from build123d import *

# Parameters (mm, degrees)
F0_R     = 11.3
F1_DEPTH = 35
F2_SIZE  = 1
F3_R     = 7.3
F4_DEPTH = 76.5
F5_SIZE2 = 20
F5_SIZE  = 2
F6_R     = 3.75
F7_DEPTH = 111.501
F8_SIZE  = 1


with BuildPart() as f1:
    # F0 (on Front) → F1 (new body)
    with BuildSketch(Plane.XZ):
        Circle(F0_R)
    extrude(amount=-F1_DEPTH)

    # F2
    f2_edges = [f1.edges().sort_by_distance(p)[0] for p in [
        (-11.3, 0, 0),
    ]]
    chamfer(f2_edges, length=F2_SIZE)

    # F3 (on face) → F4 (join)
    with BuildSketch(Plane(origin=(0, 35, 0), x_dir=(-1, 0, 0), z_dir=(0, 1, 0))):
        Circle(F3_R)
    extrude(amount=F4_DEPTH)

    # F5
    f5_edges = [f1.edges().sort_by_distance(p)[0] for p in [
        (7.3, 111.5, 0),
    ]]
    f5_side = f1.faces().sort_by_distance((0, 111.5, 0))[0]
    chamfer(f5_edges, length=F5_SIZE, length2=F5_SIZE2, reference=f5_side)

    # F6 (on face) → F7 (cut, through all)
    with BuildSketch(Plane.XZ):
        Circle(F6_R)
    extrude(amount=-F7_DEPTH, mode=Mode.SUBTRACT)

    # F8
    f8_edges = [f1.edges().sort_by_distance(p)[0] for p in [
        (-11.3, 35, 0),
    ]]
    chamfer(f8_edges, length=F8_SIZE)


solid = f1.part
Input: part model. Units: mm. Frame: model coordinates. A direction names the side the tool comes from. Coordinates: 2 decimals unless noted, no trailing zeros. Loops run counter-clockwise (first coordinate to the right, second up) from the corner with the lowest first, then second, coordinate; pieces in that order, holes last. Notation, with made-up numbers: (38, -11) -> (68, -11) arc R29 ccw to (68, 27) -> close; hole circle Ø8 at (37, 63.25). An arc over 180 degrees is marked (long way). One line per item, written item: value.
(1) Cut plane A-A (z = 0). Output: boundary loops of the cut face in (x, y).
Answer below:
outline: (-11.3, 1) -> (-10.3, 0) -> (-3.75, 0) -> (-3.75, 111.5) -> (-5.3, 111.5) -> (-7.3, 91.5) -> (-7.3, 35) -> (-10.3, 35) -> (-11.3, 34) -> close; (3.75, 0) -> (10.3, 0) -> (11.3, 1) -> (11.3, 34) -> (10.3, 35) -> (7.3, 35) -> (7.3, 91.5) -> (5.3, 111.5) -> (3.75, 111.5) -> close
(2) Pin query (flat end, axial travel): pin 1 Ø6 at (x, y) = (-8.5, 74) entering from -Z; pin 2 Ø1 at (y, z) = (85, -6) entering from -X; pin 3 Ø3 at (y, z) = (29.5, 4) entering from -X; pin 4 Ø12 at (x, z) = (0, 0) entering from +Y. Return the tip coordinate at first contact, or that it passes through.
Answer below:
pin 1: stops at z = -4.8
pin 2: stops at x = -4.8
pin 3: stops at x = -11.02
pin 4: stops at y = 111.5
(3) Draft query along X for faces 1 (the face through (-1, 111.5, 4)), 2 (the face through (-6.963, 62.854, 2.193)), 3 (the face through (-3.746, 54.97, 0.165)). Return one class per face: pulls with the +X half, pulls with the -X half, needs draft (parallel to the pull), parting line crosses it, or undercut.
Answer below:
face 1: needs draft
face 2: parting line crosses it
face 3: undercut
(4) Set-up query: faces 4 (the face through (0, 0, -4)), 5 (the face through (4, 35, -7)). Return all of +Z, -Z, +X, -X, +Y, -Y with unobstructed straight access to the full face (end or side cutting, diameter ignored); none if empty.
Answer below:
face 4: +Z, -Z, +X, -X, -Y
face 5: +Y
(5) Cut plane D-D (y = 43). Output: boundary loops of the cut face in (x, z), then the cut area to 3 significant figures.
Answer below:
outline: circle Ø14.6 at (0, 0); hole circle Ø7.5 at (0, 0)
area: 123 mm2
(6) Cut plane B-B (x = 0). Output: boundary loops of the cut face in (y, z).
Answer below:
outline: (0, -10.3) -> (1, -11.3) -> (34, -11.3) -> (35, -10.3) -> (35, -7.3) -> (91.5, -7.3) -> (111.5, -5.3) -> (111.5, -3.75) -> (0, -3.75) -> close; (0, 3.75) -> (111.5, 3.75) -> (111.5, 5.3) -> (91.5, 7.3) -> (35, 7.3) -> (35, 10.3) -> (34, 11.3) -> (1, 11.3) -> (0, 10.3) -> close
(7) Cut plane C-C (y = 104.5). Output: boundary loops of the cut face in (x, z), then the cut area to 3 significant figures.
Answer below:
outline: circle Ø12 at (0, 0); hole circle Ø7.5 at (0, 0)
area: 68.9 mm2
(8) Ray query, line 1 along Z through (x, y) = (0, 52); line 2 along Z through (x, y) = (0, 26); line 3 along Y through (x, z) = (-6, -6.75). Return the intervals inside material, ascending.
Answer below:
line 1: z = -7.3 to -3.75, 3.75 to 7.3
line 2: z = -11.3 to -3.75, 3.75 to 11.3
line 3: y = 0 to 35
